Geometry: final body of the model. Coordinates: model frame, mm. A direction names the side the tool comes from. Give positions to 0.01 mm unless a question says otherwise; leave off trailing zeros. Loops run counter-clockwise (first coordinate to the right, second up) from the corner with the lowest first, then second, coordinate; pieces in that order, holes last. Notation, with made-up numbers: M -15.5,48 L 15.5,48 A24 ccw 15.5,62 Z; hole C 79,15.25 d1. An arc over 180 degrees is marked long. Put each result on its own line as item: value.
```python
from build123d import *

# Parameters (mm, degrees)
F3_D     = 5
F3_DEPTH = 47.0757239888
F4_D     = 10


with BuildPart() as f1:
    # F0 (on Front) → F1 (revolve)
    with BuildSketch(Plane.XZ):
        Polygon((0, 0), (0, 35.6816388667), (-9.515103884, 29.1713047773), (-21.2837848812, 29.1713047773), (-23.2869647443, 19.6562018245), (-36.3076329231, 19.6562018245), (-45.071542263, 11.6434814408), (-47.0747239888, 0), align=None)
    revolve(axis=Axis((0, 0, 17.8408194333), (0, 0, -1)))

    # F3 (through all, one way)
    with BuildSketch(Plane.XZ):
        with Locations((0, 35.6816388667), (-9.515103884, 29.1713047773)):
            Circle(F3_D / 2)
    extrude(amount=-F3_DEPTH, mode=Mode.SUBTRACT)

    # F4 (through all)
    with Locations(Plane(origin=(0, 0, 0), x_dir=(1, 0, 0), z_dir=(0, 0, -1))):
        with Locations((0, 0)):
            Hole(F4_D / 2)


solid = f1.part
```
Item 1: Line query: probe 1 along Y at (x, z) = (0, 12); probe 2 along Y at (x, z) = (0, 24); probe 3 along Z at (x, y) = (-22, 15.5). Output: solid intervals per line, ascending. Write a range as [from, to].
Output values:
probe 1: [-44.68, -5], [5, 44.68]
probe 2: [-22.37, -5], [5, 22.37]
probe 3: [0, 19.66]
Item 2: Set-up query: faces 4 (the flat face through (1, -10, 0)), 5 (the flat face through (9, -4, 29.171)). Return all of +Z, -Z, +X, -X, +Y, -Y with unobstructed straight access to the full face (end or side cutting, diameter ignored); none if empty.
Output values:
face 4: -Z, +X, -X, +Y, -Y
face 5: +Z
Item 3: Pin query (flat end, axial travel): pin 1 Ø2 at (y, z) = (-10, 25) entering from -X; pin 2 Ø1 at (x, z) = (36, 9) entering from -Y; pin 3 Ø1 at (y, z) = (23.5, 6) entering from +X. Return the tip coordinate at first contact, or that it passes through.
Output values:
pin 1: x = -20.31
pin 2: y = -28.52
pin 3: x = 39.9
Item 4: Section A-A on x = 0. Output: boundary loops of the cut face in (y, z), then the cut area to 3 significant figures.
Output values:
outline: M -47.07,0 L -5,0 L -5,32.26 L -9.52,29.17 L -21.28,29.17 L -23.29,19.66 L -36.31,19.66 L -45.07,11.64 Z; M 5,0 L 47.07,0 L 45.07,11.64 L 36.31,19.66 L 23.29,19.66 L 21.28,29.17 L 9.52,29.17 L 5,32.26 Z
area: 1,870 mm²
Item 5: Mould query, pull axis X, two halves, no side actions, for faces 1 (the cylindrical face through (1.08, 4.88, 16.36)), 2 (the conical face through (-20.856, -40.097, 10.915)), 3 (the flat face through (-1, -24, 19.656)). Classes: pulls with the +X half, pulls with the -X half, needs draft (parallel to the pull), parting line crosses it, or undercut.
Output values:
face 1: undercut
face 2: parting line crosses it
face 3: needs draft
Item 6: Section B-B on z = 23. Output: boundary loops of the cut face in (x, y).
Output values:
outline: C 0,0 d45.17; hole C 0,0 d10
Item 7: Section C-C on z = 9. Output: boundary loops of the cut face in (x, y), then the cut area to 3 significant figures.
Output values:
outline: C 0,0 d91.05; hole C 0,0 d10
area: 6,430 mm²
